```python
from build123d import *

# Parameters (mm, degrees)
F2_R     = 3.571875
F3_DEPTH = 6.35


with BuildPart() as f1:
    # F0 (on Front) → F1 (revolve)
    with BuildSketch(Plane.XZ):
        with BuildLine():
            Line((5.953125, 6.35), (0, 6.35))
            Line((0, 6.35), (0, 0))
            Line((0, 0), (12.7, 0))
            Line((12.7, 0), (12.7, 12.7))
            ThreePointArc((12.7, 12.7), (12.235032, 13.822532), (11.1125, 14.2875))
            Line((11.1125, 14.2875), (8.334375, 14.2875))
            ThreePointArc((8.334375, 14.2875), (7.211843, 13.822532), (6.746875, 12.7))
            Line((6.746875, 12.7), (6.746875, 7.14375))
            ThreePointArc((6.746875, 7.14375), (6.514391, 6.582484), (5.953125, 6.35))
        make_face()
    revolve(axis=Axis((0, 0, 3.175), (0, 0, -1)))

    # F2 (on face) → F3 (cut, through all)
    with BuildSketch(Plane.XY.offset(6.35)):
        Circle(F2_R)
    extrude(amount=-F3_DEPTH, mode=Mode.SUBTRACT)


solid = f1.part
```
CAD build for the part. Positions are in the model's coordinates, mm. A direction names the side the tool comes from. Coordinates: 2 decimals unless noted, no trailing zeros. Order: outer loops, then holes, each group sorted by start corner. A loop starts at its lowest first (then second) coordinate and runs counter-clockwise, first axis right, second up. Notation, with made-up numbers: M 52.5,-36 L 106.5,-36 A12 ccw 106.5,-24 Z; hole C -38,-15 d5. An arc over 180 degrees is marked long. Write each question's results on one line, items separated by ' | '. Start each with the question number.
Q1. Cut at C-C (z = 12.25). List the corners of the cut face in (x, y), then the cut area to 3 significant figures.
Q2. Drill centre lines: probe 1 along Y at (x, z) = (0, 4.5); probe 2 along Y at (x, z) = (0, 8.65). Where is each one in solid material? Low to high. Write a range as from..to.
Q3. Pull direction Y, two halves, no side cores. Call faces 1 (the cylindrical face through (-2.75, 12.4, 6.44)), 2 (the flat face through (-3, 3, 0)), 3 (the flat face through (3, 3, 6.35)): +Y half, -Y half, draft (parallel to the pull), parting line (faces both ways), or undercut.
Q4. Which spindle directions (+Z, -Z, +X, -X, +Y, -Y) get a long thin tool onto all of the face, cutting with end or side? Do faces 4 (the flat face through (4.1, -7.5, 14.288)), 5 (the cylindrical face through (-4.97, -4.56, 9.88)). Say none if no direction does.
Q5. Flat gauge pins, fed straight in: P1, Ø1, axis at x = -10, z = 11, coming from the -Y side; P2, Ø13, axis at x = 1, y = 2.5, coming from the +Z side; P3, Ø1, axis at y = 7.5, z = 9.5, coming from the -X side; P4, Ø5, axis at x = 9, z = 6.5, coming from the +Y side. Where does each tip first touch, or does it go through?
Found:
1) outline: C 0,0 d25.4; hole C 0,0 d13.49 | area: 364 mm²
2) probe 1: -12.7..-3.57, 3.57..12.7 | probe 2: -12.7..-6.75, 6.75..12.7
3) face 1: parting line | face 2: draft | face 3: undercut
4) face 4: +Z, +X, -X, +Y, -Y | face 5: +Z
5) P1: y = -8.43 | P2: z = 14.29 | P3: x = -10.6 | P4: y = 10.91
